Source: CAD feature listing. Evaluate the final solid. Frame: model axes, mm. A direction names the side the tool comes from. Round coordinates to 2 decimals unless told otherwise and drop trailing zeros. Write each loop counter-clockwise with the first axis right and the second up, starting at its lowest first coordinate (ties: lowest second). Pieces come first, ordered by that corner, then holes. Notation, with made-up numbers: (-9.5, 6) -> (21.5, 6) arc R10 ccw to (21.5, 15) -> close; hole circle Ø10 at (28, -3). An arc over 180 degrees is marked (long way). Put each result on its own line as item: value.
```python
from build123d import *

# Parameters (mm, degrees)
SKETCH1_R                = 76.2
BOSS_EXTRUDE1_DEPTH      = 3.175
BOSS_EXTRUDE2_DEPTH      = 3.175
SKETCH3_R                = 4
BOSS_EXTRUDE3_DEPTH      = 12.954
BOSS_EXTRUDE3_DEPTH_BACK = 6.35


with BuildPart() as part:
    # Sketch1 → Boss-Extrude1 (new body)
    with BuildSketch(Plane(origin=(0, 0, 0), x_dir=(1, 0, 0), z_dir=(0, 1, 0))):
        Circle(SKETCH1_R)
    extrude(amount=BOSS_EXTRUDE1_DEPTH)

    # Sketch2 → Boss-Extrude2 (add)
    with BuildSketch(Plane(origin=(0, 3.175, 0), x_dir=(1, 0, 0), z_dir=(0, 1, 0))):
        with BuildLine():
            Line((-74.7395, 1.4605), (74.7395, 1.4605))
            ThreePointArc((74.7395, 1.4605), (76.2, 0), (74.7395, -1.4605))
            Line((74.7395, -1.4605), (-74.7395, -1.4605))
            ThreePointArc((-74.7395, -1.4605), (-76.2, 0), (-74.7395, 1.4605))
        make_face()
        with BuildLine():
            Line((1.4605, 74.7395), (1.4605, -74.7395))
            ThreePointArc((1.4605, -74.7395), (0, -76.2), (-1.4605, -74.7395))
            Line((-1.4605, -74.7395), (-1.4605, 74.7395))
            ThreePointArc((-1.4605, 74.7395), (0, 76.2), (1.4605, 74.7395))
        make_face()
    extrude(amount=BOSS_EXTRUDE2_DEPTH)

    # Sketch3 → Boss-Extrude3 (add, two sides)
    with BuildSketch(Plane(origin=(0, 6.35, 0), x_dir=(1, 0, 0), z_dir=(0, 1, 0))) as boss_extrude3_sk:
        Circle(SKETCH3_R)
    extrude(amount=BOSS_EXTRUDE3_DEPTH)
    extrude(boss_extrude3_sk.sketch, amount=-BOSS_EXTRUDE3_DEPTH_BACK)


solid = part.part
```
Q1. Cut plane C-C on y = 14.25. Output: boundary loops of the cut face in (x, z).
Ans:
outline: circle Ø8 at (0, 0)
Q2. Material intervals for line 1 (Y direction, x = -55, z = 9) (3 decimals); line 2 (X direction, y = 2, z = 2); line 3 (Z direction, x = 41.5, y = 5.25), sorted ascending. Write a range as [from, to].
Ans:
line 1: y = [0, 3.175]
line 2: x = [-76.17, 76.17]
line 3: z = [-1.46, 1.46]
Q3. Reachability of faces 1 (the flat face through (0, 19.304, 0)), 2 (the flat face through (29, 3.175, -30)), 3 (the flat face through (-30, 3.175, -30)), 4 (the flat face through (-30, 3.175, 29)), 5 (the flat face through (29, 3.175, 29)) from +Z, -Z, +X, -X, +Y, -Y: full face, straight path, thin tool, end or side. Return the list, or none.
Ans:
face 1: +Z, -Z, +X, -X, +Y
face 2: -Z, +X, +Y
face 3: -Z, -X, +Y
face 4: +Z, -X, +Y
face 5: +Z, +X, +Y
Q4. Pin query (flat end, axial travel): pin 1 (23 mm diameter, centred on x = -41, z = 50, fed in from +Y) (3 decimals); pin 2 (1.6 mm diameter, centred on x = 31.5, y = 5.5, fed in from +Z); pin 3 (1 mm diameter, centred on y = 8, z = 25, fed in from -X); pin 4 (3.5 mm diameter, centred on y = 4.5, z = 37, fed in from -X). Return the tip coordinate at first contact, or that it passes through.
Ans:
pin 1: stops at y = 3.175
pin 2: stops at z = 1.46
pin 3: passes through
pin 4: stops at x = -67.24
